Build history of the part. All positions in model axes, mm. Round coordinates to 2 decimals unless told otherwise and drop trailing zeros. Write each loop counter-clockwise with the first axis right and the second up, starting at its lowest first coordinate (ties: lowest second). Pieces come first, ordered by that corner, then holes. Notation, with made-up numbers: M 48.25,12.25 L 63.25,12.25 A35 ccw 63.25,48.25 Z; hole C -12.5,10.25 d3. An arc over 180 degrees is marked long. Write item = value, one per line. Start each with the question number.
Q1. Drop flat-ended pins along their axis: P1, Ø2, axis at x = -11, y = 1, coming from the -Z side; P2, Ø1.8, axis at x = -135, y = 2.5, coming from the +Z side; P3, Ø1.8, axis at y = 3, z = -5.5, coming from the +X side. Give the stop position or say it passes through.
Q2. Band-saw the part on C-C on x = -149. Write the cut outline in (y, z).
Q3. Band-saw the part on B-B on y = 4.65. Write the cut outline in (x, z).
Q4. Band-saw the part on D-D on x = -36.5. Write the cut outline in (y, z).
Q5. Band-saw the part on A-A on z = -65.5. Write the cut outline in (x, y), plus the area to 3 significant figures.
Q6. Probe L1, parallel to X at y = 1.2, z = -17.5; L2, parallel to X at y = 3.5, z = -29.5; L3, parallel to Z at x = -127, y = 4.95. List the from-to ranges inside material, lowest first.
```python
from build123d import *

# Parameters (mm, degrees)
SKETCH1_W           = 10
SKETCH1_H           = 6
BOSS_EXTRUDE1_DEPTH = 6


with BuildPart() as part:
    # Sketch1 → Boss-Extrude1 (new body)
    with BuildSketch(Plane(origin=(0, 0, 0), x_dir=(1, 0, 0), z_dir=(0, 1, 0))):
        with BuildLine():
            Line((0, 9.722175855), (-7.5, 9.722175855))
            Line((-7.5, 9.722175855), (-7.5, 21.194984734))
            ThreePointArc((-7.5, 21.194984734), (-9.890826257, 27.683472612), (-15.920094989, 31.069391053))
            Line((-15.920094989, 31.069391053), (-120.920094989, 47.869391053))
            ThreePointArc((-120.920094989, 47.869391053), (-128.988487878, 45.604158477), (-132.5, 37.994984734))
            Line((-132.5, 37.994984734), (-132.5, 9.722175855))
            Line((-132.5, 9.722175855), (-140, 9.722175855))
            Line((-140, 9.722175855), (-140, 3.722175855))
            Line((-140, 3.722175855), (-155.5, 3.722175855))
            Line((-155.5, 3.722175855), (-155.5, 9.722175855))
            Line((-155.5, 9.722175855), (-163, 9.722175855))
            Line((-163, 9.722175855), (-163, 71.03416911))
            ThreePointArc((-163, 71.03416911), (-157.389342775, 82.732042518), (-144.754634366, 85.678881532))
            Line((-144.754634366, 85.678881532), (5.745365634, 52.327080978))
            ThreePointArc((5.745365634, 52.327080978), (14.197873407, 47.071711331), (17.5, 37.682368556))
            Line((17.5, 37.682368556), (17.5, 9.722175855))
            Line((17.5, 9.722175855), (10, 9.722175855))
            Line((10, 9.722175855), (10, 3.722175855))
            Line((10, 3.722175855), (0, 3.722175855))
            Line((0, 3.722175855), (0, 9.722175855))
        make_face()
        with Locations((-147.75, 66.722175855)):
            Rectangle(SKETCH1_W, SKETCH1_H, mode=Mode.SUBTRACT)
    extrude(amount=BOSS_EXTRUDE1_DEPTH)


solid = part.part
```
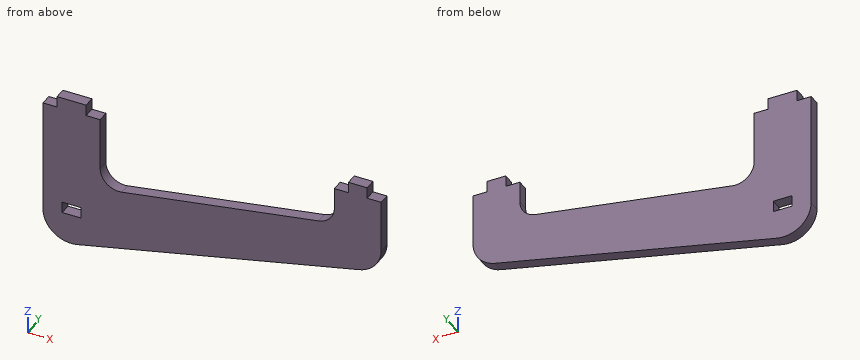
Conclusion:
q1.P1 = -56.26
q1.P2 = -9.72
q1.P3 = 10
q2.outline = M 0,-86 L 6,-86 L 6,-69.72 L 0,-69.72 Z; M 0,-63.72 L 6,-63.72 L 6,-3.72 L 0,-3.72 Z
q3.outline = M -163,-71.03 A15 ccw -144.75,-85.68 L 5.75,-52.33 A15 ccw 17.5,-37.68 L 17.5,-9.72 L 10,-9.72 L 10,-3.72 L 0,-3.72 L 0,-9.72 L -7.5,-9.72 L -7.5,-21.19 A10 cw -15.92,-31.07 L -120.92,-47.87 A10 cw -132.5,-37.99 L -132.5,-9.72 L -140,-9.72 L -140,-3.72 L -155.5,-3.72 L -155.5,-9.72 L -163,-9.72 Z; hole M -152.75,-69.72 L -142.75,-69.72 L -142.75,-63.72 L -152.75,-63.72 Z
q4.outline = M 0,-61.69 L 6,-61.69 L 6,-34.36 L 0,-34.36 Z
q5.outline = M -163,0 L -152.75,0 L -152.75,6 L -163,6 Z; M -142.75,0 L -53.7,0 L -53.7,6 L -142.75,6 Z
q5.area = 596 mm^2
q6.L1 = -163 to -132.5, -7.5 to 17.5
q6.L2 = -163 to -132.5, -11.93 to 17.5
q6.L3 = -81.74 to -46.93
